Geometry: see drawing. Coordinates: mm, zero at the bounding-box minimum. Give positions to 0.01 mm unless a question says otherwise; leave off trailing zeros. Write each loop counter-clockwise with the first axis right and the second up, starting at its lowest first coordinate (ties: lowest second). Pieces come first, ordered by that corner, then holes. Notation, with made-up numbers: M -20,-5.75 L 29,-5.75 A8 cw 29,6.25 Z; hole C 51,63.5 d4. An arc over 180 degrees is marked long. Use a Markdown table: item, result. Add a question column.
1) Pin query (flat end, axial travel): pin 1 (9 mm diameter, centred on x = 599.5, z = 5, fed in from -Y). Return the tip coordinate at first contact, or that it passes through.
2) Section C-C on z = 4.5. Return the cut outline in (x, y), then the cut area to 3 significant figures.
3) Section B-B on x = 310. Return the cut outline in (y, z).
4) Line query: line 1 (Y direction, x = 310, z = 8.25); line 2 (X direction, y = 51, z = 12.75); line 3 (X direction, y = 23, z = 3.25). Output: solid intervals per line, ascending.
5) Section A-A on y = 65. Return the cut outline in (x, z).
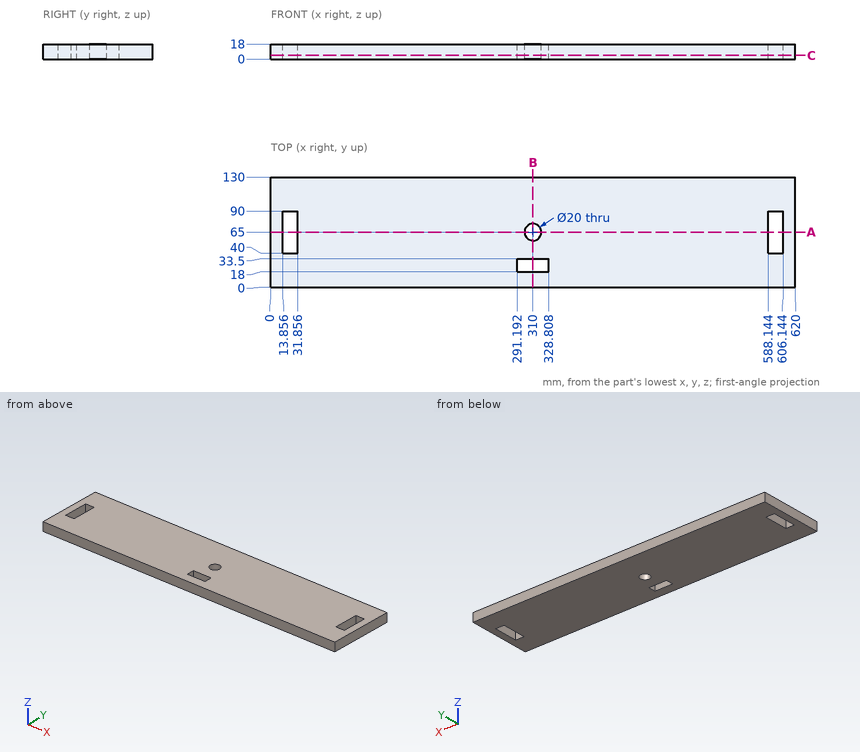
Found:
| question | item | result |
|---|---|---|
| 1 | pin 1 | y = 0 |
| 2 | outline | M 0,0 L 620,0 L 620,130 L 0,130 Z; hole M 13.86,40 L 31.86,40 L 31.86,90 L 13.86,90 Z; hole M 291.19,18 L 328.81,18 L 328.81,33.5 L 291.19,33.5 Z; hole C 310,65 d20; hole M 588.14,40 L 606.14,40 L 606.14,90 L 588.14,90 Z |
| 2 | area | 77,900 mm² |
| 3 | outline | M 0,0 L 18,0 L 18,18 L 0,18 Z; M 33.5,0 L 55,0 L 55,18 L 33.5,18 Z; M 75,0 L 130,0 L 130,18 L 75,18 Z |
| 4 | line 1 | 0 to 18, 33.5 to 55, 75 to 130 |
| 4 | line 2 | 0 to 13.86, 31.86 to 588.14, 606.14 to 620 |
| 4 | line 3 | 0 to 291.19, 328.81 to 620 |
| 5 | outline | M 0,0 L 13.86,0 L 13.86,18 L 0,18 Z; M 31.86,0 L 300,0 L 300,18 L 31.86,18 Z; M 320,0 L 588.14,0 L 588.14,18 L 320,18 Z; M 606.14,0 L 620,0 L 620,18 L 606.14,18 Z |
